Verification items for the finished model (mm, model axes). Face numbers are marked on the shaded views. A direction names the side the tool comes from. Coordinates: 2 decimals unless noted, no trailing zeros. Order: outer loops, then holes, each group sorted by start corner. A loop starts at its lowest first (then second) coordinate and runs counter-clockwise, first axis right, second up. Notation, with made-up numbers: M -24,-19.75 L 18,-19.75 A28 ccw 18,9.25 Z; hole C 49.25,-25 d10. An arc over 180 degrees is marked long. Answer as a JSON object with one key per item and string values. Group by question number.
(1) Cross-section at C-C (x = 28). Enter the section's corners in (y, z), plus the area to 3 significant figures.
(2) Cross-section at A-A (z = 7.5). Enter the section's corners in (x, y) (3 decimals), plus the area to 3 significant figures.
(3) Cross-section at D-D (x = 12.5). Enter the section's corners in (y, z).
(4) Access from +Z, -Z, +X, -X, +Y, -Y to the whole of each face (thin tool, end or side, straight path). Record for the marked faces 1, 2 and 3.
(5) Mould release check, pull along X, two halves, no side actions. Record for the marked faces 4, 5, 6 and 7: released by +X, released by -X, zero draft, split by the parting line, or undercut.
(6) Gauge pin test, flat ends, axial feed: pin 1 Ø3 at (y, z) = (-4.5, 13.5) entering from -X (3 decimals); pin 2 Ø2 at (y, z) = (-43.5, 5) entering from -X; pin 3 Ø5 at (y, z) = (-23.5, 13) entering from +X (3 decimals); pin 4 Ø16 at (x, y) = (33.16, -40.43) entering from -Z. Record the tip position at first contact, or that the pin passes through.
(7) Material ranges on line 1 (Z direction, x = 33.5, y = 23); line 2 (X direction, y = -1, z = 3.75) (3 decimals); line 3 (X direction, y = 19.5, z = 4.5), recorded low to high.
(8) Cross-section at B-B (y = -35). Enter the section's corners in (x, z) (3 decimals).
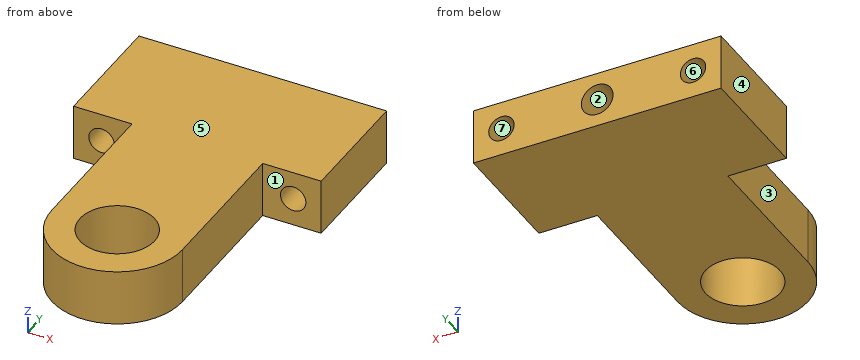
from build123d import *

# Parameters (mm, degrees)
SKETCH1_R           = 10
BOSS_EXTRUDE1_DEPTH = 15
SKETCH2_R           = 3.4
CUT_EXTRUDE1_DEPTH  = 54
SKETCH3_R           = 4.25
CUT_EXTRUDE2_DEPTH  = 28


with BuildPart() as part:
    # Sketch1 → Boss-Extrude1 (new body)
    with BuildSketch(Plane.XY):
        with BuildLine():
            Line((0, 0), (0, 33))
            Line((0, 33), (66.33, 33))
            Line((66.33, 33), (66.33, 0))
            Line((66.33, 0), (50.665, 0))
            Line((50.665, 0), (50.665, -40.433566532))
            ThreePointArc((50.665, -40.433566532), (33.165, -57.933566532), (15.665, -40.433566532))
            Line((15.665, -40.433566532), (15.665, 0))
            Line((15.665, 0), (0, 0))
        make_face()
        with Locations((33.165, -40.433566532)):
            Circle(SKETCH1_R, mode=Mode.SUBTRACT)
    extrude(amount=BOSS_EXTRUDE1_DEPTH)

    # Sketch2 → Cut-Extrude1 (cut)
    with BuildSketch(Plane(origin=(0, 33, 0), x_dir=(1, 0, 0), z_dir=(0, 1, 0))):
        with Locations(Location((58.831, -7.5, 0), (0, 0, 270))):
            Circle(SKETCH2_R)
        with Locations(Location((7.499, -7.5, 0), (0, 0, 180))):
            Circle(SKETCH2_R)
    extrude(amount=-CUT_EXTRUDE1_DEPTH, mode=Mode.SUBTRACT)

    # Sketch3 → Cut-Extrude2 (cut)
    with BuildSketch(Plane(origin=(0, 33, 0), x_dir=(1, 0, 0), z_dir=(0, 1, 0))):
        with Locations(Location((33.165, -7.5, 0), (0, 0, 270))):
            Circle(SKETCH3_R)
    extrude(amount=-CUT_EXTRUDE2_DEPTH, mode=Mode.SUBTRACT)


solid = part.part
Taken from the geometry:
{
 "1": {"outline": "M -57.15,0 L -49,0 L -49,15 L -57.15,15 Z; M -31.87,0 L 33,0 L 33,15 L -31.87,15 Z", "area": "1,100 mm²"},
 "2": {"outline": "M 0,0 L 4.099,0 L 4.099,33 L 0,33 Z; M 10.899,0 L 15.665,0 L 15.665,-40.434 A17.5 ccw 50.665,-40.434 L 50.665,0 L 55.431,0 L 55.431,33 L 37.415,33 L 37.415,5 L 28.915,5 L 28.915,33 L 10.899,33 Z; M 62.231,0 L 66.33,0 L 66.33,33 L 62.231,33 Z; hole C 33.165,-40.434 d20", "area": "3,080 mm²"},
 "3": {"outline": "M 0,0 L 33,0 L 33,15 L 0,15 Z"},
 "4": {"face 1": "+Z, -Z, +X, -Y", "face 2": "+Y", "face 3": "+Z, -Z, -X, -Y"},
 "5": {"face 4": "released by -X", "face 5": "zero draft", "face 6": "undercut", "face 7": "undercut"},
 "6": {"pin 1": "stops at x = 15.665", "pin 2": "stops at x = 15.79", "pin 3": "stops at x = 50.665", "pin 4": "passes through"},
 "7": {"line 1": "z = 0 to 3.26, 11.74 to 15", "line 2": "x = 15.665 to 50.665", "line 3": "x = 0 to 5.9, 9.1 to 30.15, 36.18 to 57.23, 60.43 to 66.33"},
 "8": {"outline": "M 15.665,0 L 24.77,0 L 24.77,15 L 15.665,15 Z; M 41.56,0 L 50.665,0 L 50.665,15 L 41.56,15 Z"}
}
